```python
from build123d import *

# Parameters (mm, degrees)
ESTRUSIONE_ESTRUSIONE1_DEPTH = 15
SCHIZZO2_R                   = 2.75
TAGLIO_ESTRUSIONE1_DEPTH     = 15
SCHIZZO3_R                   = 1.5
TAGLIO_ESTRUSIONE2_DEPTH     = 15


with BuildPart() as part:
    # Schizzo1 → Estrusione-Estrusione1 (new body)
    with BuildSketch(Plane.XY):
        Polygon((0, 0), (-30, 0), (-30, 50), (-28, 50), (-28, 2), (0, 2), align=None)
    extrude(amount=ESTRUSIONE_ESTRUSIONE1_DEPTH)

    # Schizzo2 → Taglio-Estrusione1 (cut)
    with BuildSketch(Plane.ZY.offset(30)):
        with Locations((7.5, 44)):
            Circle(SCHIZZO2_R)
        with Locations((7.5, 16)):
            Circle(SCHIZZO2_R)
    extrude(amount=-TAGLIO_ESTRUSIONE1_DEPTH, mode=Mode.SUBTRACT)

    # Schizzo3 → Taglio-Estrusione2 (cut)
    with BuildSketch(Plane.XZ):
        with Locations((-6, 7.5)):
            Circle(SCHIZZO3_R)
        with Locations((-15, 7.5)):
            Circle(SCHIZZO3_R)
    extrude(amount=-TAGLIO_ESTRUSIONE2_DEPTH, mode=Mode.SUBTRACT)


solid = part.part
```
For this review, take the finished solid that the model builds, in its own axes (mm). A direction names the side the tool comes from. Round coordinates to 2 decimals unless told otherwise and drop trailing zeros. Loops run counter-clockwise (first coordinate to the right, second up) from the corner with the lowest first, then second, coordinate; pieces in that order, holes last.
(1) We need section A-A (y = 44). Give the boundary of the cut face in (x, z).
Returned:
outline: (-30, 0) - (-28, 0) - (-28, 4.75) - (-30, 4.75) - close; (-30, 10.25) - (-28, 10.25) - (-28, 15) - (-30, 15) - close
(2) We need section C-C (z = 7.5). Give the boundary of the cut face in (x, y).
Returned:
outline: (-30, 0) - (-16.5, 0) - (-16.5, 2) - (-28, 2) - (-28, 13.25) - (-30, 13.25) - close; (-30, 18.75) - (-28, 18.75) - (-28, 41.25) - (-30, 41.25) - close; (-30, 46.75) - (-28, 46.75) - (-28, 50) - (-30, 50) - close; (-13.5, 0) - (-7.5, 0) - (-7.5, 2) - (-13.5, 2) - close; (-4.5, 0) - (0, 0) - (0, 2) - (-4.5, 2) - close
(3) Tool access review of faces 1 (the flat face through (-29, 50, 7)), 2 (the flat face through (-28, 26, 7)): name each direction out of +Z, -Z, +X, -X, +Y, -Y from which nothing blocks a thin tool from reaching the whole face with its end or side.
Returned:
face 1: +Z, -Z, +X, -X, +Y
face 2: +Z, -Z, +X, +Y
(4) Clearance check with flat-ended pins moving along their axes: P1, Ø1.8, axis at x = -6, z = 7.5, coming from the -Y side; P2, Ø1.5, axis at y = 14.5, z = 11.5, coming from the +X side; P3, Ø4, axis at x = -22, z = 8.5, coming from the -Y side; P4, Ø7.5, axis at x = -11.5, z = 10, coming from the +Y side. State where each tip first meets the part, or that it passes through.
Returned:
P1: passes through
P2: stops at x = -28
P3: stops at y = 0
P4: stops at y = 2
(5) We need section B-B (x = -15). Give the boundary of the cut face in (y, z), plus the area to 3 significant figures.
Returned:
outline: (0, 0) - (2, 0) - (2, 6) - (0, 6) - close; (0, 9) - (2, 9) - (2, 15) - (0, 15) - close
area: 24.0 mm2
(6) Wall thickness on line 1 along Z through (x, y) = (-15, 0.8); line 2 along Y through (x, z) = (-29.3, 7.5); line 3 along X through (y, z) = (13, 4.75): over which ranges is each line inside the solid? List them lowest first.
Returned:
line 1: z = 0 to 6, 9 to 15
line 2: y = 0 to 13.25, 18.75 to 41.25, 46.75 to 50
line 3: x = -30 to -28
(7) Mouldability with a two-part tool opening along X and no side actions: class faces 3 (the cylindrical face through (-29.014, 46.727, 7.142)), 4 (the flat face through (0, 1, 7)), 5 (the cylindrical face through (-6, 1, 6)), 6 (the cylindrical face through (-16.2, 1, 6.6)) as released by +X, released by -X, zero draft, split by the parting line, or undercut.
Returned:
face 3: zero draft
face 4: released by +X
face 5: undercut
face 6: undercut
(8) We need section D-D (z = 3.75). Give the boundary of the cut face in (x, y), plus the area to 3 significant figures.
Returned:
outline: (-30, 0) - (0, 0) - (0, 2) - (-28, 2) - (-28, 50) - (-30, 50) - close
area: 156 mm2
